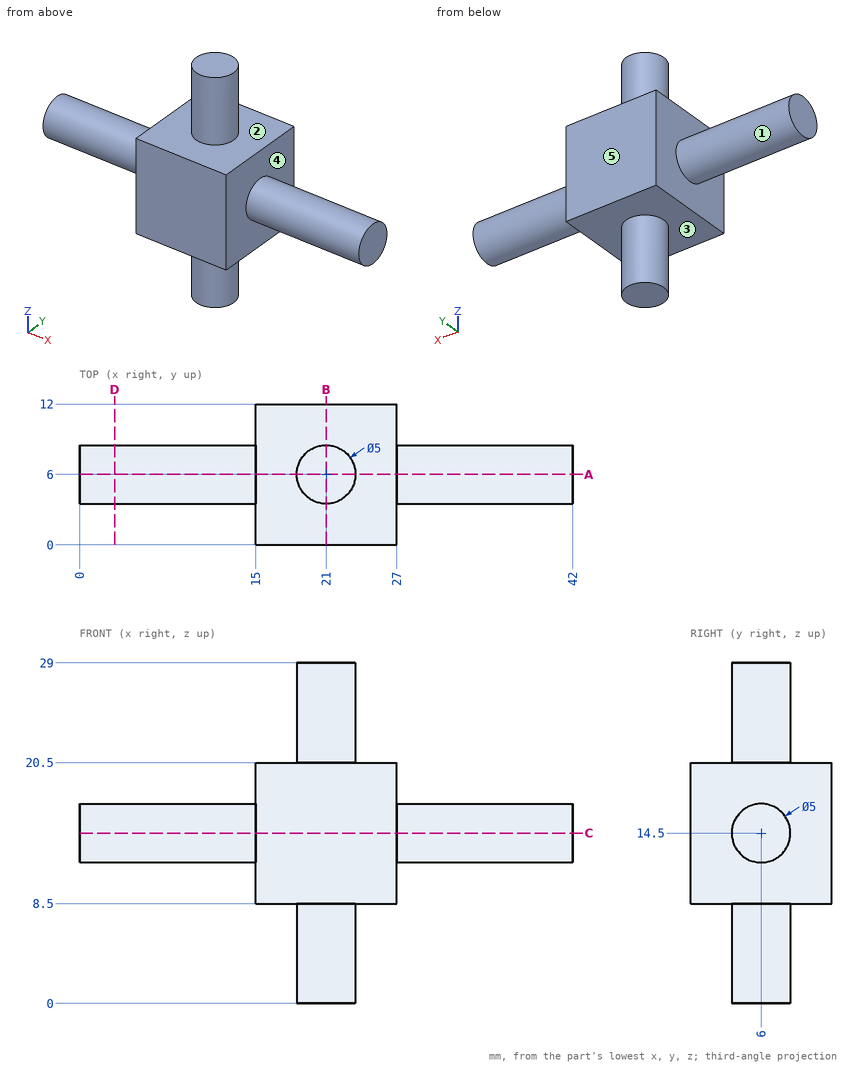
Geometry: see drawing. Coordinates: mm, zero at the bounding-box minimum. A direction names the side the tool comes from. Give positions to 0.01 mm unless a question says otherwise; leave off trailing zeros. Write each loop counter-clockwise with the first axis right and the second up, starting at its lowest first coordinate (ties: lowest second). Pieces come first, ordered by that corner, then holes. Notation, with made-up numbers: (62, 65) - (88, 65) arc R17 ccw to (88, 70) - close; hole circle Ø7 at (-38.5, 44.25). An arc over 180 degrees is marked (long way). Return JSON: item names as keys, results as strings. Group by question number.
1) Line query: line 1 (X direction, y = 8.5, z = 10.5); line 2 (Z direction, x = 23, y = 1.25); line 3 (Z direction, x = 33.5, y = 6). Output: solid intervals per line, ascending.
2) Section C-C on z = 14.5. Return the cut outline in (x, y), plus the area to 3 significant figures.
3) Section D-D on x = 3. Return the cut outline in (y, z).
4) Section B-B on x = 21. Return the cut outline in (y, z).
5) Set-up query: the marked faces 1, 2, 3, 4 and 5. Return all of +Z, -Z, +X, -X, +Y, -Y with unobstructed straight access to the full face (end or side cutting, diameter ignored); none if empty.
6) Section A-A on y = 6. Return the cut outline in (x, z).
7) First-contact query: P1, Ø12, axis at x = 37, z = 15.5, coming from the +Y side; P2, Ø6, axis at x = 23, z = 5, coming from the -Y side. Flat tips, straight axial feed; report the tip coordinate or a pass-through.
Filled in:
{
 "1": {"line 1": "x = 15 to 27", "line 2": "z = 8.5 to 20.5", "line 3": "z = 12 to 17"},
 "2": {"outline": "(0, 3.5) - (15, 3.5) - (15, 0) - (27, 0) - (27, 3.5) - (42, 3.5) - (42, 8.5) - (27, 8.5) - (27, 12) - (15, 12) - (15, 8.5) - (0, 8.5) - close", "area": "294 mm^2"},
 "3": {"outline": "circle Ø5 at (6, 14.5)"},
 "4": {"outline": "(0, 8.5) - (3.5, 8.5) - (3.5, 0) - (8.5, 0) - (8.5, 8.5) - (12, 8.5) - (12, 20.5) - (8.5, 20.5) - (8.5, 29) - (3.5, 29) - (3.5, 20.5) - (0, 20.5) - close"},
 "5": {"face 1": "-X", "face 2": "+Z", "face 3": "-Z", "face 4": "+X", "face 5": "+Z, -Z, +X, -X, +Y"},
 "6": {"outline": "(0, 12) - (15, 12) - (15, 8.5) - (18.5, 8.5) - (18.5, 0) - (23.5, 0) - (23.5, 8.5) - (27, 8.5) - (27, 12) - (42, 12) - (42, 17) - (27, 17) - (27, 20.5) - (23.5, 20.5) - (23.5, 29) - (18.5, 29) - (18.5, 20.5) - (15, 20.5) - (15, 17) - (0, 17) - close"},
 "7": {"P1": "stops at y = 8.5", "P2": "stops at y = 3.5"}
}
